```python
from build123d import *

# Parameters (mm, degrees)
F0_R     = 9.6012
F1_DEPTH = 11.684
F2_W     = 5.08
F2_H     = 7
F3_DEPTH = 25.4


with BuildPart() as f1:
    # F0 (on Top) → F1 (new body)
    with BuildSketch(Plane.XY):
        with BuildLine():
            ThreePointArc((11.914125, -4.398138), (61.122967, 0), (11.914125, 4.398138))
            ThreePointArc((11.914125, 4.398138), (-12.7, 0), (11.914125, -4.398138))
        make_face()
        Circle(F0_R, mode=Mode.SUBTRACT)
    extrude(amount=F1_DEPTH)

    # F2 (on face) → F3 (cut)
    with BuildSketch(Plane(origin=(0, 0, 0), x_dir=(1, 0, 0), z_dir=(0, 0, -1))):
        with Locations((27.342967, 0.609253)):
            Rectangle(F2_W, F2_H)
        with Locations((48.422967, 0.609253)):
            Rectangle(F2_W, F2_H)
    extrude(amount=-F3_DEPTH, mode=Mode.SUBTRACT)


solid = f1.part
```
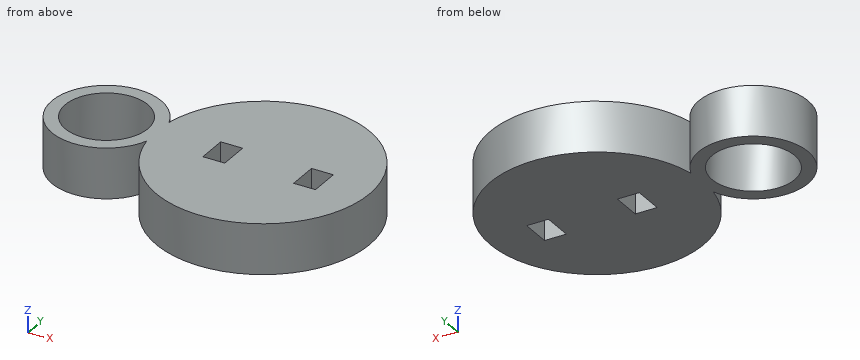
CAD build for the part. Positions are in the model's coordinates, mm. Coordinates: 2 decimals unless noted, no trailing zeros. Write each loop counter-clockwise with the first axis right and the second up, starting at its lowest first coordinate (ties: lowest second). Pieces come first, ordered by that corner, then holes. Notation, with made-up numbers: (67.25, 74) -> (112.25, 74) arc R5 cw to (112.25, 82) -> close; hole circle Ø3 at (42, 34). An arc over 180 degrees is marked (long way). Use CSV: the item, a comma, the result in double quotes. Start each with the question number.
Item 1: Band-saw the part on B-B, the plane x = 0. Write the cut outline in (y, z), plus the area to 3 significant figures.
Item 2: Band-saw the part on A-A, the plane y = 0. Write the cut outline in (x, z).
Item 3: Drop flat-ended pins along their axis: P1, Ø2.5, axis at x = 27.5, z = 4.5, coming from the -Y side; P2, Ø1.5, axis at x = 49.5, z = 7, coming from the +Y side; P3, Ø4, axis at x = 48.5, z = 6.5, coming from the -Y side; P4, Ø15.5, axis at x = 0, y = 0, coming from the -Z side. Give the stop position or say it passes through.
Item 4: Band-saw the part on C-C, the plane z = 2. Write the cut outline in (x, y), plus the area to 3 significant figures.
Item 5: Band-saw the part on D-D, the plane x = 7.5. Write the cut outline in (y, z), plus the area to 3 significant figures.
Item 6: Wall check: probe 1 along Y at (x, z) = (0, 3.75); probe 2 along X at (y, z) = (2, 10.5); probe 3 along X at (y, z) = (-1, 1.5). Give the ranges that are in metal, low to high.
Response values:
1,outline,"(-12.7, 0) -> (-9.6, 0) -> (-9.6, 11.68) -> (-12.7, 11.68) -> close; (9.6, 0) -> (12.7, 0) -> (12.7, 11.68) -> (9.6, 11.68) -> close"
1,area,"72.4 mm2"
2,outline,"(-12.7, 0) -> (-9.6, 0) -> (-9.6, 11.68) -> (-12.7, 11.68) -> close; (9.6, 0) -> (24.8, 0) -> (24.8, 11.68) -> (9.6, 11.68) -> close; (29.88, 0) -> (45.88, 0) -> (45.88, 11.68) -> (29.88, 11.68) -> close; (50.96, 0) -> (61.12, 0) -> (61.12, 11.68) -> (50.96, 11.68) -> close"
3,P1,"stops at y = -23.62"
3,P2,"stops at y = 21.46"
3,P3,"stops at y = -22.62"
3,P4,"passes through"
4,outline,"(11.91, -4.4) arc R24.8 ccw (long way) to (11.91, 4.4) arc R12.7 ccw (long way) to start; hole circle Ø19.2 at (0, 0); hole (24.8, -4.11) -> (29.88, -4.11) -> (29.88, 2.89) -> (24.8, 2.89) -> close; hole (45.88, -4.11) -> (50.96, -4.11) -> (50.96, 2.89) -> (45.88, 2.89) -> close"
4,area,"2,070 mm2"
5,outline,"(-10.25, 0) -> (-5.99, 0) -> (-5.99, 11.68) -> (-10.25, 11.68) -> close; (5.99, 0) -> (10.25, 0) -> (10.25, 11.68) -> (5.99, 11.68) -> close"
5,area,"99.4 mm2"
6,probe 1,"y = -12.7 to -9.6, 9.6 to 12.7"
6,probe 2,"x = -12.54 to -9.39, 9.39 to 24.8, 29.88 to 45.88, 50.96 to 61.04"
6,probe 3,"x = -12.66 to -9.55, 9.55 to 24.8, 29.88 to 45.88, 50.96 to 61.1"
